Geometry check sheet. Reference: the model listing, model coordinates, mm. Face numbers are marked on the shaded views. A direction names the side the tool comes from. Give positions to 0.01 mm unless a question says otherwise; leave off trailing zeros. Write each loop counter-clockwise with the first axis right and the second up, starting at its lowest first coordinate (ties: lowest second). Pieces come first, ordered by that corner, then holes.
(1) Thickness scan on line 1 along Y through (x, z) = (-4.5, 62); line 2 along Z through (x, y) = (-18, -14.5); line 3 along X through (y, z) = (35.5, 38.5). Record the ranges inside material, lowest first.
(2) Cross-section at D-D (y = -5.5). Record the boundary of the cut face in (x, z).
(3) Cross-section at C-C (x = 118). Record the boundary of the cut face in (y, z).
(4) Cross-section at A-A (z = 34). Record the boundary of the cut face in (x, y), and give its area (3 significant figures).
(5) Depth check by flat-ended pin: P1, Ø5, axis at x = 17.5, z = 29.5, coming from the +Y side; P2, Ø10, axis at x = 55, y = 23.5, coming from the +Z side; P3, Ø3, axis at x = 93, y = 25.5, coming from the +Z side. Enter the tip coordinate at first touch or a pass-through.
(6) Tool access check on the marked faces 1, 2 and 3. Record the directions out of +Z, -Z, +X, -X, +Y, -Y that give a thin tool (end or side, any length) a straight path to the whole face; none if there is none.
(7) Cross-section at B-B (y = 18). Record the boundary of the cut face in (x, z).
```python
from build123d import *

# Parameters (mm, degrees)
F0_W      = 185.4944750667
F0_H      = 110.638756305
F1_DEPTH  = 25
F2_SIZE   = 5
F3_W      = 31.4006619155
F3_H      = 26.9978269935
F3_W_2    = 41.5280163288
F3_H_2    = 18.5919255018
F4_DEPTH  = 25
F4_FACE_W = 41.5280163288
F4_FACE_H = 18.5919255018
F5_ANGLE  = 30
F6_R      = 5


with BuildPart() as f1:
    # F0 (on Top) → F1 (new body)
    with BuildSketch(Plane.XY):
        with Locations((57.9323507845, 20.6255745143)):
            Rectangle(F0_W, F0_H)
    extrude(amount=F1_DEPTH)

    # F2
    f2_edges = [f1.edges().sort_by_distance(p)[0] for p in [
        (57.932351, -34.693804, 25),
        (-34.814887, 20.625575, 25),
        (150.679588, 20.625575, 25),
        (150.679588, 20.625575, 0),
    ]]
    chamfer(f2_edges, length=F2_SIZE)

    # F3 (on face) → F4 (join)
    with BuildSketch(Plane.XY.offset(25)):
        with Locations((74.988739565, 13.4989134967)):
            Rectangle(F3_W, F3_H)
        with Locations((8.6979772896, 43.5124337673)):
            Rectangle(F3_W_2, F3_H_2)
    extrude(amount=F4_DEPTH)

    # F4_face (on face) → F5 (revolve)
    with BuildSketch(Plane(origin=(8.6979772896, 43.5124337673, 50), x_dir=(1, 0, 0), z_dir=(0, 0, 1))):
        Rectangle(F4_FACE_W, F4_FACE_H)
    revolve(axis=Axis((29.461985454, 43.5124337673, 50), (0, 1, 0)), revolution_arc=F5_ANGLE)

    # F6
    f6_edges = [f1.edges().sort_by_distance(p)[0] for p in [
        (11.479827, 34.216471, 60.382004),
        (11.479827, 52.808397, 60.382004),
        (29.461985, 43.512434, 50),
    ]]
    fillet(f6_edges, radius=F6_R)


solid = f1.part
```
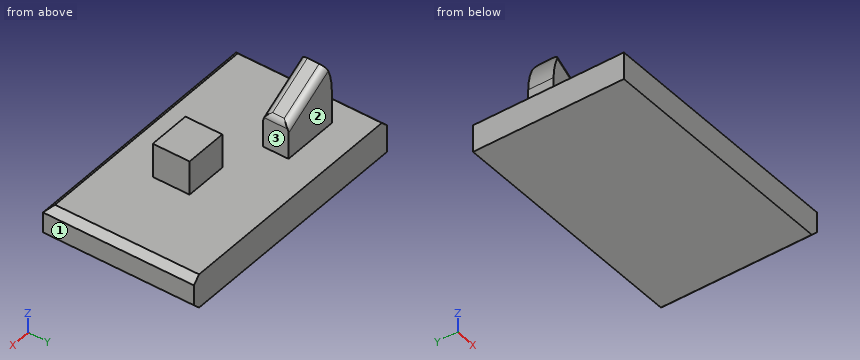
Reply:
1. line 1: y = 34.22 to 52.81
1. line 2: z = 0 to 25
1. line 3: x = -12.07 to 29.46
2. outline: (-34.81, 0) - (145.68, 0) - (150.68, 5) - (150.68, 20) - (145.68, 25) - (-29.81, 25) - (-34.81, 20) - close
3. outline: (-34.69, 0) - (75.94, 0) - (75.94, 25) - (-29.69, 25) - (-34.69, 20) - close
4. outline: (-12.07, 34.22) - (29.46, 34.22) - (29.46, 52.81) - (-12.07, 52.81) - close; (59.29, 0) - (90.69, 0) - (90.69, 27) - (59.29, 27) - close
4. area: 1,620 mm2
5. P1: stops at y = 52.81
5. P2: stops at z = 50
5. P3: stops at z = 25
6. face 1: +Z, -Z, +X, +Y, -Y
6. face 2: +Z, +X, -X, +Y
6. face 3: +Z, +X, +Y, -Y
7. outline: (-34.81, 0) - (145.68, 0) - (150.68, 5) - (150.68, 20) - (145.68, 25) - (90.69, 25) - (90.69, 50) - (59.29, 50) - (59.29, 25) - (-29.81, 25) - (-34.81, 20) - close
